from build123d import *

# Parameters (mm, degrees)
CUT_EXTRUDE1_DEPTH      = 205.091015236
CUT_EXTRUDE1_DEPTH_BACK = 205.091015236
SKETCH2_R               = 1.778


with BuildPart() as part:
    # Sketch1 → Revolve1 (revolve)
    with BuildSketch(Plane(origin=(0, 0, 0), x_dir=(0, 0, -1), z_dir=(1, 0, 0)), mode=Mode.PRIVATE) as revolve1_sk:
        Polygon((0, 36.5125), (196.85, 36.5125), (196.85, 37.084), (196.07039578, 38.1), (0, 38.1), align=None)
    revolve(revolve1_sk.sketch.rotate(Axis((0, 0, 6.983722976), (0, 0, -1)), 90), axis=Axis((0, 0, 6.983722976), (0, 0, -1)))

    # Sketch2 → Cut-Extrude1 (cut, two sides: drawn at the far end of the back side and taken through both)
    with BuildSketch(Plane(origin=(0, 0, 0), x_dir=(0, 0, -1), z_dir=(1, 0, 0)).offset(-CUT_EXTRUDE1_DEPTH_BACK)):
        with Locations((5.08, 0)):
            Circle(SKETCH2_R)
    extrude(amount=CUT_EXTRUDE1_DEPTH + CUT_EXTRUDE1_DEPTH_BACK, mode=Mode.SUBTRACT)


solid = part.part
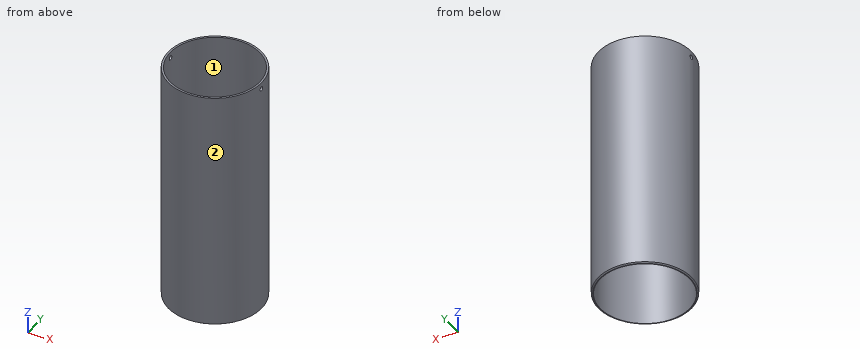
Build history of the part. All positions in model axes, mm. Face numbers are marked on the shaded views. Round coordinates to 2 decimals unless told otherwise and drop trailing zeros. Loops run counter-clockwise (first coordinate to the right, second up) from the corner with the lowest first, then second, coordinate; pieces in that order, holes last. Notation, with made-up numbers: (40.25, 39.5) -> (46.25, 39.5) arc R16 cw to (46.25, 58.5) -> close; hole circle Ø9 at (33.5, 0.25). An arc over 180 degrees is marked (long way). One line per item, written item: value. Start each with the question number.
Q1. Drop flat-ended pins along their axis: pin 1 Ø4 at (y, z) = (17, -140.5) entering from -X; pin 2 Ø1.5 at (y, z) = (9, -81.5) entering from -X; pin 3 Ø10 at (x, z) = (17.5, -22.5) entering from -Y; pin 4 Ø4 at (y, z) = (0, -5.08) entering from +X. Give the stop position or say it passes through.
Q2. Probe line 1 along X through (y, z) = (-1, -107); line 2 along Y through (x, z) = (0, -50); line 3 along X through (y, z) = (-29, -44.5). List the from-to ranges inside material, lowest first.
Q3. Two-plate mould, pull along X, no slides. Class the marked faces 1 and 2: released by +X, released by -X, zero draft, split by the parting line, or undercut.
Q4. Cut at B-B on z = -184.5. List the corners of the cut face in (x, y) (1 decimal), plus the area to 3 significant figures.
Q5. Cut at A-A on x = 0. List the corners of the cut face in (y, z).
Computed:
1. pin 1: x = -35.02
1. pin 2: x = -37.2
1. pin 3: y = -35.99
1. pin 4: x = 38.1
2. line 1: -38.09 to -36.5, 36.5 to 38.09
2. line 2: -38.1 to -36.51, 36.51 to 38.1
2. line 3: -24.71 to -22.18, 22.18 to 24.71
3. face 1: undercut
3. face 2: split by the parting line
4. outline: circle Ø76.2 at (0, 0); hole circle Ø73 at (0, 0)
4. area: 372 mm²
5. outline: (-38.1, -196.07) -> (-37.08, -196.85) -> (-36.51, -196.85) -> (-36.51, 0) -> (-38.1, 0) -> close; (36.51, -196.85) -> (37.08, -196.85) -> (38.1, -196.07) -> (38.1, 0) -> (36.51, 0) -> close
